Check sheet for the modelled part. Datum: model origin and axes. Units: mm. Give positions to 0.01 mm unless a question says otherwise; leave off trailing zeros. Loops run counter-clockwise (first coordinate to the right, second up) from the corner with the lowest first, then second, coordinate; pieces in that order, holes last. Notation, with made-up numbers: (-3, 73.5) - (27, 73.5) arc R14 ccw to (27, 82.5) - close; hole circle Ø11 at (-2, 29). An arc over 180 degrees is marked (long way). Answer in a Markdown table with one row per item. Add a question column.
(1) Thickness scan on L1, parallel to Y at x = 180, z = 2.75; L2, parallel to X at y = 4.25, z = 7; L3, parallel to X at y = -8.25, z = 1.25. Record the ranges inside material, lowest first.
(2) Go/stop test with flat-tipped pins: P1, Ø6, axis at y = -5, z = 9, coming from the -X side; P2, Ø1.5, axis at y = 7, z = 7, coming from the -X side; P3, Ø2, axis at y = 4.5, z = 2.5, coming from the -X side; P4, Ø18, axis at x = 180, y = 0, coming from the -Z side. Record where each tip stops, or that it passes through.
(3) Sectioned sample at A-A on x = 180. Enter the section's corners in (y, z), then the cut area to 3 significant figures.
(4) Sectioned sample at B-B on z = 2.5. Enter the section's corners in (x, y), then the cut area to 3 significant figures.
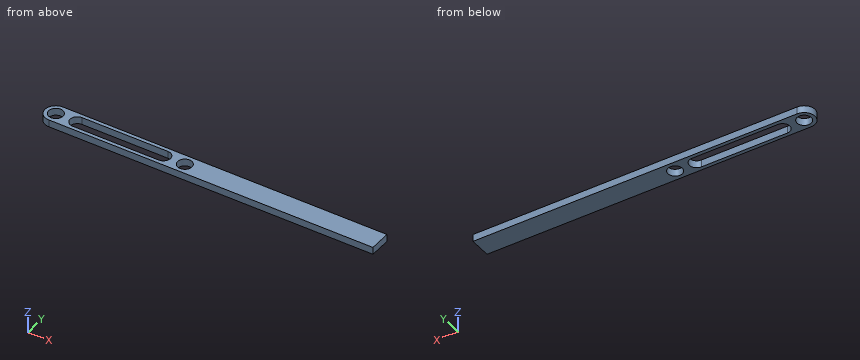
from build123d import *

# Parameters (mm, degrees)
SKETCH1_R           = 10
BOSS_EXTRUDE1_DEPTH = 10


with BuildPart() as part:
    # Sketch1 → Boss-Extrude1 (new body)
    with BuildSketch(Plane.XY):
        with BuildLine():
            Line((0, 15), (180, 15))
            Line((180, 15), (452.334951872, 15))
            Line((452.334951872, 15), (452.334951872, -15))
            Line((452.334951872, -15), (180, -15))
            Line((180, -15), (0, -15))
            ThreePointArc((0, -15), (-15, 0), (0, 15))
        make_face()
        Circle(SKETCH1_R, mode=Mode.SUBTRACT)
        with Locations((180, 0)):
            Circle(SKETCH1_R, mode=Mode.SUBTRACT)
        with BuildLine():
            Line((30, 10), (150, 10))
            ThreePointArc((150, 10), (160, 0), (150, -10))
            Line((150, -10), (30, -10))
            ThreePointArc((30, -10), (20, 0), (30, 10))
        make_face(mode=Mode.SUBTRACT)
    extrude(amount=BOSS_EXTRUDE1_DEPTH)


solid = part.part
Reply:
| question | item | result |
|---|---|---|
| 1 | L1 | -15 to -10, 10 to 15 |
| 1 | L2 | -14.39 to -9.05, 9.05 to 20.95, 159.05 to 170.95, 189.05 to 452.33 |
| 1 | L3 | -12.53 to -5.65, 5.65 to 24.35, 155.65 to 174.35, 185.65 to 452.33 |
| 2 | P1 | x = -14.87 |
| 2 | P2 | x = -13.64 |
| 2 | P3 | x = -14.59 |
| 2 | P4 | through |
| 3 | outline | (-15, 0) - (-10, 0) - (-10, 10) - (-15, 10) - close; (10, 0) - (15, 0) - (15, 10) - (10, 10) - close |
| 3 | area | 100 mm^2 |
| 4 | outline | (0, -15) - (452.33, -15) - (452.33, 15) - (0, 15) arc R15 ccw to start; hole circle Ø20 at (0, 0); hole (30, -10) - (150, -10) arc R10 ccw to (150, 10) - (30, 10) arc R10 ccw to start; hole circle Ø20 at (180, 0) |
| 4 | area | 10,600 mm^2 |
